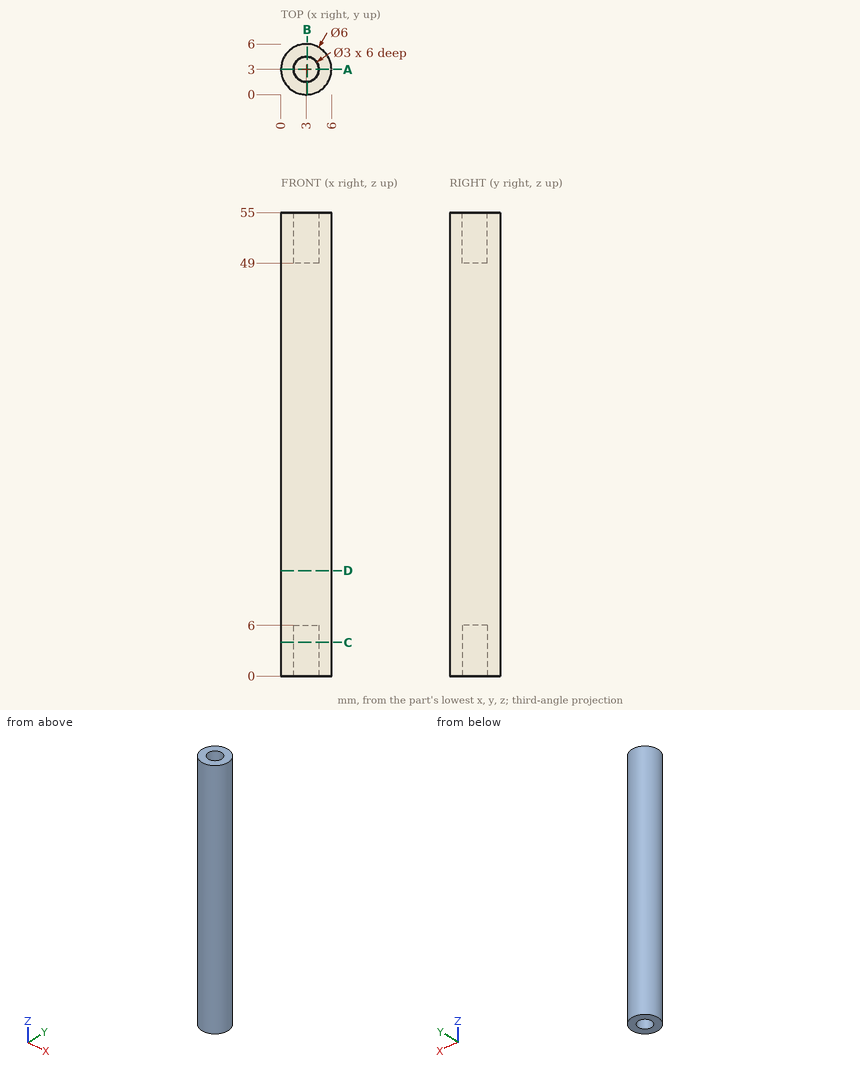
Source: three-view drawing plus pictorial views. Frame: mm from the lowest corner of the part. Give positions to 0.01 mm unless a question says otherwise; leave off trailing zeros. Loops run counter-clockwise (first coordinate to the right, second up) from the corner with the lowest first, then second, coordinate; pieces in that order, holes last.
1) Section query C-C on z = 4. Return the cut outline in (x, y), and give its area (3 significant figures).
A:
outline: circle Ø6 at (3, 3); hole circle Ø3 at (3, 3)
area: 21.2 mm2
2) Section query A-A on y = 3. Return the cut outline in (x, z), and give its area (3 significant figures).
A:
outline: (0, 0) - (1.5, 0) - (1.5, 6) - (4.5, 6) - (4.5, 0) - (6, 0) - (6, 55) - (4.5, 55) - (4.5, 49) - (1.5, 49) - (1.5, 55) - (0, 55) - close
area: 294 mm2
3) Line query: L1, parallel to Y at x = 3, z = 50.45; L2, parallel to Z at x = 2.4, y = 2.4; L3, parallel to Y at x = 2.75, z = 28.5. Output: solid intervals per line, ascending.
A:
L1: y = 0 to 1.5, 4.5 to 6
L2: z = 6 to 49
L3: y = 0.01 to 5.99
4) Section query D-D on z = 12.5. Return the cut outline in (x, y).
A:
outline: circle Ø6 at (3, 3)
5) Contact query for flat-ended pins moving along their axis: pin 1 (2.5 mm diameter, centred on x = 3, y = 3, fed in from +Z); pin 2 (2.5 mm diameter, centred on x = 3, y = 3, fed in from -Z); pin 3 (2 mm diameter, centred on x = 1, z = 36.5, fed in from +Y). Output: stop coordinate, or through.
A:
pin 1: stops at z = 49
pin 2: stops at z = 6
pin 3: stops at y = 5.83
